Print and shaded views of the part. All mm, measured from the part's lowest x, y and z. Round coordinates to 2 decimals unless told otherwise and drop trailing zeros. Loops run counter-clockwise (first coordinate to the right, second up) from the corner with the lowest first, then second, coordinate; pieces in that order, holes last. Notation, with made-up numbers: (66.5, 15) -> (109.5, 15) arc R15 cw to (109.5, 42) -> close; hole circle Ø2 at (52, 48.25). An arc over 180 degrees is marked (long way). Answer as CSV lines item,"result".
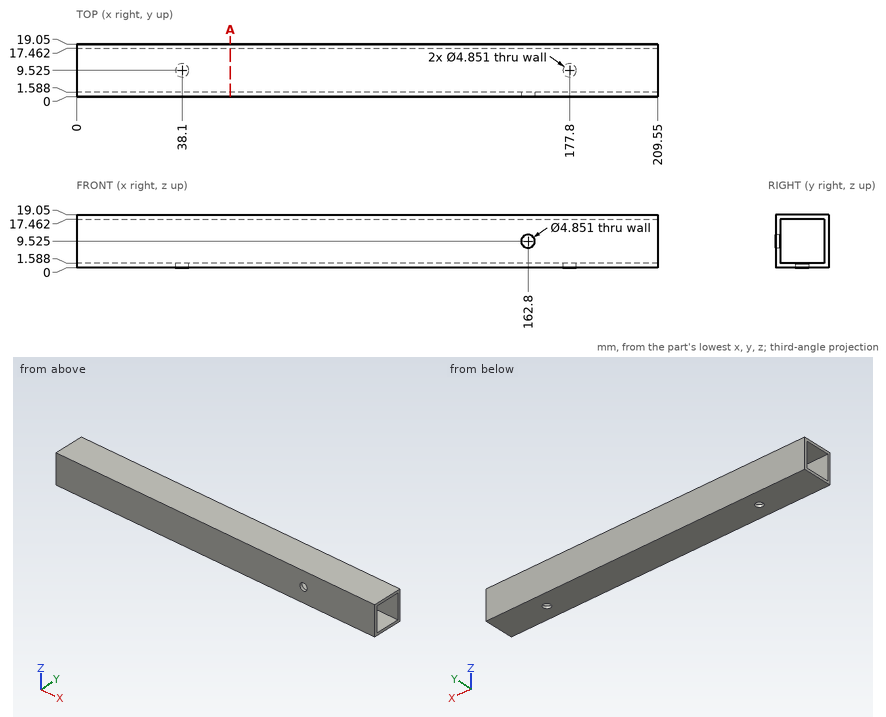
Q1. Saw through at A-A, the plane x = 55.5. Write the cut outline in (y, z), then the cut area to 3 significant figures.
Geometry results:
outline,"(0, 0) -> (19.05, 0) -> (19.05, 19.05) -> (0, 19.05) -> close; hole (1.59, 1.59) -> (17.46, 1.59) -> (17.46, 17.46) -> (1.59, 17.46) -> close"
area,"111 mm2"
Q2. Drop flat-ended pins along their axis: P1, Ø8, axis at y = 13, z = 10.5, coming from the -X side; P2, Ø3, axis at x = 177.8, y = 9.525, coming from the -Z side. Give the stop position or say it passes through.
Geometry results:
P1,"through"
P2,"z = 17.46"
Q3. Drill centre lines: line 1 along Z through (x, y) = (198.5, 12.75); line 2 along Y through (x, z) = (177.8, 1). Where is each one in solid material? Low to high.
Geometry results:
line 1,"0 to 1.59, 17.46 to 19.05"
line 2,"0 to 7.1, 11.95 to 19.05"
